from build123d import *

# Parameters (mm, degrees)
SKETCH1_R           = 34.5
BOSS_EXTRUDE1_DEPTH = 5
BOSS_EXTRUDE2_START = 7.5
SKETCH4_R           = 34.5
SKETCH4_R_2         = 31.5
BOSS_EXTRUDE2_DEPTH = 7.5
SKETCH5_R           = 3
CUT_EXTRUDE1_DEPTH  = 50.363448016
SKETCH6_R           = 3
CUT_EXTRUDE2_DEPTH  = 2
SKETCH8_R           = 1.6
CUT_EXTRUDE3_DEPTH  = 50.363448016
BOSS_EXTRUDE3_START = 7.5
BOSS_EXTRUDE3_DEPTH = 7.5
CIRPATTERN1_COUNT   = 16
SKETCH10_R          = 11.5
CUT_EXTRUDE4_DEPTH  = 2
BOSS_EXTRUDE4_START = 8.5
SKETCH11_R          = 34.5
SKETCH11_R_2        = 33
BOSS_EXTRUDE4_DEPTH = 8.5
BOSS_EXTRUDE5_START = -21
BOSS_EXTRUDE5_DEPTH = 21
SKETCH15_R          = 1.6
CUT_EXTRUDE5_DEPTH  = 15
CIRPATTERN2_COUNT   = 8
SKETCH16_R          = 2
CUT_EXTRUDE6_DEPTH  = 59.107658703


with BuildPart() as part:
    # Sketch1 → Boss-Extrude1 (new body)
    with BuildSketch(Plane(origin=(0, 0, 0), x_dir=(1, 0, 0), z_dir=(0, 1, 0))):
        with Locations(Location((0, 0, 0), (0, 0, 270))):
            Circle(SKETCH1_R)
    extrude(amount=-BOSS_EXTRUDE1_DEPTH)

    # Sketch4 → Boss-Extrude2 (add)
    with BuildSketch(Plane(origin=(0, 0, 0), x_dir=(1, 0, 0), z_dir=(0, 1, 0)).offset(BOSS_EXTRUDE2_START)):
        with Locations(Location((0, 0, 0), (0, 0, 270))):
            Circle(SKETCH4_R)
        with Locations(Location((0, 0, 0), (0, 0, 270))):
            Circle(SKETCH4_R_2, mode=Mode.SUBTRACT)
    extrude(amount=-BOSS_EXTRUDE2_DEPTH)

    # Sketch5 → Cut-Extrude1 (cut, through all)
    with BuildSketch(Plane(origin=(0, 0, 0), x_dir=(1, 0, 0), z_dir=(0, 1, 0))):
        with Locations(Location((0, 0, 0), (0, 0, 270))):
            Circle(SKETCH5_R)
    extrude(amount=-CUT_EXTRUDE1_DEPTH, mode=Mode.SUBTRACT)

    # Sketch6 → Cut-Extrude2 (cut)
    with BuildSketch(Plane(origin=(0, 0, 0), x_dir=(1, 0, 0), z_dir=(0, 1, 0))):
        with Locations(Location((-15.5, 15.5, 0), (0, 0, 270))):
            Circle(SKETCH6_R)
        with Locations(Location((15.5, 15.5, 0), (0, 0, 270))):
            Circle(SKETCH6_R)
        with Locations(Location((15.5, -15.5, 0), (0, 0, 270))):
            Circle(SKETCH6_R)
        with Locations(Location((-15.5, -15.5, 0), (0, 0, 270))):
            Circle(SKETCH6_R)
    extrude(amount=-CUT_EXTRUDE2_DEPTH, mode=Mode.SUBTRACT)

    # Sketch8 → Cut-Extrude3 (cut, through all)
    with BuildSketch(Plane(origin=(0, 0, 0), x_dir=(1, 0, 0), z_dir=(0, 1, 0))):
        with Locations(Location((-15.5, 15.5, 0), (0, 0, 270))):
            Circle(SKETCH8_R)
        with Locations(Location((15.5, 15.5, 0), (0, 0, 270))):
            Circle(SKETCH8_R)
        with Locations(Location((15.5, -15.5, 0), (0, 0, 270))):
            Circle(SKETCH8_R)
        with Locations(Location((-15.5, -15.5, 0), (0, 0, 270))):
            Circle(SKETCH8_R)
    extrude(amount=-CUT_EXTRUDE3_DEPTH, mode=Mode.SUBTRACT)

    # Sketch9 → Boss-Extrude3 (add)
    with BuildSketch(Plane(origin=(0, 0, 0), x_dir=(1, 0, 0), z_dir=(0, 1, 0)).offset(BOSS_EXTRUDE3_START)):
        with BuildLine():
            ThreePointArc((-4.810876836, 31.130458783), (0, 28.5), (4.810876836, 31.130458783))
            ThreePointArc((4.810876836, 31.130458783), (0, 31.5), (-4.810876836, 31.130458783))
        make_face()
    boss_extrude3 = extrude(amount=-BOSS_EXTRUDE3_DEPTH)

    # CirPattern1: Boss-Extrude3 ×16 about axis
    cirpattern1_axis = Axis((0, 0, 0), (0, 1, 0))
    for i in range(1, CIRPATTERN1_COUNT):
        add(boss_extrude3.rotate(cirpattern1_axis, i * 360 / CIRPATTERN1_COUNT))

    # Sketch10 → Cut-Extrude4 (cut)
    with BuildSketch(Plane(origin=(0, -5, 0), x_dir=(-1, 0, 0), z_dir=(0, -1, 0))):
        with Locations(Location((0, 0, 0), (0, 0, 90))):
            Circle(SKETCH10_R)
    extrude(amount=-CUT_EXTRUDE4_DEPTH, mode=Mode.SUBTRACT)

    # Sketch11 → Boss-Extrude4 (add)
    with BuildSketch(Plane(origin=(0, 7.5, 0), x_dir=(1, 0, 0), z_dir=(0, 1, 0)).offset(BOSS_EXTRUDE4_START)):
        with Locations(Location((0, 0, 0), (0, 0, 270))):
            Circle(SKETCH11_R)
        with Locations(Location((0, 0, 0), (0, 0, 270))):
            Circle(SKETCH11_R_2, mode=Mode.SUBTRACT)
    extrude(amount=-BOSS_EXTRUDE4_DEPTH)

    # Sketch12 → Boss-Extrude5 (add)
    with BuildSketch(Plane.XZ.offset(5).offset(BOSS_EXTRUDE5_START)):
        with BuildLine():
            ThreePointArc((-4.986855227, 34.137681159), (0, 34.5), (4.986855227, 34.137681159))
            ThreePointArc((4.986855227, 34.137681159), (0, 39.5), (-4.986855227, 34.137681159))
        make_face()
    boss_extrude5 = extrude(amount=BOSS_EXTRUDE5_DEPTH)

    # Sketch15 → Cut-Extrude5 (cut)
    with BuildSketch(Plane(origin=(0, 16, 0), x_dir=(1, 0, 0), z_dir=(0, 1, 0))):
        with Locations(Location((0, -36, 0), (0, 0, 270))):
            Circle(SKETCH15_R)
    cut_extrude5 = extrude(amount=-CUT_EXTRUDE5_DEPTH, mode=Mode.SUBTRACT)

    # CirPattern2: Boss-Extrude5, Cut-Extrude5 ×8 about axis
    cirpattern2_axis = Axis((0, 0, 0), (0, 1, 0))
    add([boss_extrude5.rotate(cirpattern2_axis, i * 360 / CIRPATTERN2_COUNT) for i in range(1, CIRPATTERN2_COUNT)])
    add([cut_extrude5.rotate(cirpattern2_axis, i * 360 / CIRPATTERN2_COUNT) for i in range(1, CIRPATTERN2_COUNT)], mode=Mode.SUBTRACT)

    # Sketch16 → Cut-Extrude6 (cut, through all)
    with BuildSketch(Plane(origin=(0, 0, 0), x_dir=(1, 0, 0), z_dir=(0, 1, 0))):
        with Locations(Location((0, 22.5, 0), (0, 0, 270))):
            Circle(SKETCH16_R)
    extrude(amount=-CUT_EXTRUDE6_DEPTH, mode=Mode.SUBTRACT)


solid = part.part
Can you work these out from the model? Positions are in its coordinate system, mm. A direction names the side the tool comes from. Round coordinates to 2 decimals unless told otherwise and drop trailing zeros. Loops run counter-clockwise (first coordinate to the right, second up) from the corner with the lowest first, then second, coordinate; pieces in that order, holes last. Notation, with made-up numbers: (-38.5, 21) - (4.5, 21) arc R17 ccw to (4.5, 47) - close; hole circle Ø8 at (36.5, 11.5). An arc over 180 degrees is marked (long way). Use CSV: the item, a comma, the result in double quotes. Start each with the question number.
1) If we section it at A-A on x = 0: Count the separate pieces of the cut face and the enclosed holes in it, plus the area to 4 significant figures.
2) If we section it at B-B on z = 0: Write out the boundary of the cut face in (x, y).
3) For pin 1 Ø8 at (y, z) = (-0.5, -7) entering from +X; pin 2 Ø8 at (x, z) = (15.5, 15.5) entering from +Y; pin 3 Ø8 at (x, y) = (-16, 4.5) entering from -Z, each with a flat end and sliding along its axis, tell me the tip position at first contact or that it passes through.
4) Please list where these lines run through material, in increasing order: probe 1 along X at (y, z) = (12, 24.5); probe 2 along Y at (x, z) = (-4, -16.5); probe 3 along X at (y, z) = (14.5, -12). Write a range as [from, to].
5) If we section it at D-D on z = 10: Write out the boundary of the cut face in (x, y).
6) For faces 3 (the cylindrical face through (16.58, -3.48, 14.32)), 4 (the cylindrical face through (-13.09, 5.65, -31.92)), 5 (the cylindrical face through (-6.16, 3.8, 30.89)), 6 (the cylindrical face through (-31.92, 5.65, 13.09)), which set-ups out of +Z, -Z, +X, -X, +Y, -Y let a thin tool reach every point of the face, with its end or its side?
7) We'd pull the mould along Z, two halves only. Please class faces 1 (the cylindrical face through (26.18, 3.8, 17.52)), 2 (the cylindrical face through (13.31, 5.65, -31.83)): released by +Z, released by -Z, zero draft, split by the parting line, or undercut.
Geometry results:
1,separate pieces,"3"
1,enclosed holes,"0"
1,area,"490.5 mm2"
2,outline,"(-39.5, -5) - (-11.5, -5) - (-11.5, -3) - (-3, -3) - (-3, 0) - (-28.5, 0) - (-28.5, 7.5) - (-33, 7.5) - (-33, 16) - (-34.4, 16) - (-34.4, 1) - (-37.6, 1) - (-37.6, 16) - (-39.5, 16) - close; (3, -3) - (11.5, -3) - (11.5, -5) - (39.5, -5) - (39.5, 16) - (37.6, 16) - (37.6, 1) - (34.4, 1) - (34.4, 16) - (33, 16) - (33, 7.5) - (28.5, 7.5) - (28.5, 0) - (3, 0) - close"
3,pin 1,"stops at x = 38.5"
3,pin 2,"stops at y = 0"
3,pin 3,"stops at z = -32.35"
4,probe 1,"x = [-29.39, -26.74], [-24.17, -22.11], [22.11, 24.17], [26.74, 29.39]"
4,probe 2,"y = [-5, 0]"
4,probe 3,"x = [-32.35, -30.74], [30.74, 32.35]"
5,outline,"(-33.02, -5) - (-5.68, -5) - (-5.68, -3) - (5.68, -3) - (5.68, -5) - (33.02, -5) - (33.02, 16) - (31.45, 16) - (31.45, 7.5) - (26.81, 7.5) - (26.81, 0) - (-26.81, 0) - (-26.81, 7.5) - (-31.45, 7.5) - (-31.45, 16) - (-33.02, 16) - close"
6,face 3,"+Y, -Y"
6,face 4,"-Z, +Y, -Y"
6,face 5,"+Y"
6,face 6,"-X, +Y, -Y"
7,face 1,"undercut"
7,face 2,"released by -Z"
